```python
from build123d import *

# Parameters (mm, degrees)
F1_DEPTH      = 5.08
F2_START      = -15.494
F2_DEPTH      = 4.826
F3_DEPTH      = 15.748
F3_DEPTH_BACK = 1.016


with BuildPart() as f1:
    # F0 (on Front) → F1 (new body)
    with BuildSketch(Plane.XZ):
        with BuildLine():
            Line((-50.7880747318, 53.6880129844), (-50.7880747318, 47.4713742733))
            Line((-50.7880747318, 47.4713742733), (0, 13.6126577854))
            ThreePointArc((0, 13.6126577854), (30.4237649591, -0.4397436147), (63.6866472612, -4.5209346608))
            Line((63.6866472612, -4.5209346608), (63.7305527925, 0))
            ThreePointArc((63.7305527925, 0), (33.6220207616, 3.8020605731), (5.8134317271, 15.9536753451))
            ThreePointArc((5.8134317271, 15.9536753451), (2.8748778359, 17.8437288794), (0, 19.8292964965))
            Line((0, 19.8292964965), (-50.7880747318, 53.6880129844))
        make_face()
        with BuildLine():
            Line((-50.7880747318, 47.4713742733), (-50.7880747318, -22.5119870156))
            Line((-50.7880747318, -22.5119870156), (63.5119252682, -22.5119870156))
            Line((63.5119252682, -22.5119870156), (63.6866472612, -4.5209346608))
            ThreePointArc((63.6866472612, -4.5209346608), (30.4237649591, -0.4397436147), (0, 13.6126577854))
            Line((0, 13.6126577854), (-50.7880747318, 47.4713742733))
        make_face()
    extrude(amount=F1_DEPTH)



with BuildPart() as f2:
    # F0 (on Front) → F2 (new body)
    with BuildSketch(Plane.XZ.offset(F2_START)):
        with BuildLine():
            Line((-50.7880747318, 47.4713742733), (-50.7880747318, -22.5119870156))
            Line((-50.7880747318, -22.5119870156), (63.5119252682, -22.5119870156))
            Line((63.5119252682, -22.5119870156), (63.6866472612, -4.5209346608))
            ThreePointArc((63.6866472612, -4.5209346608), (30.4237649591, -0.4397436147), (0, 13.6126577854))
            Line((0, 13.6126577854), (-50.7880747318, 47.4713742733))
        make_face()
        with BuildLine():
            Line((-50.7880747318, 53.6880129844), (-50.7880747318, 47.4713742733))
            Line((-50.7880747318, 47.4713742733), (0, 13.6126577854))
            ThreePointArc((0, 13.6126577854), (30.4237649591, -0.4397436147), (63.6866472612, -4.5209346608))
            Line((63.6866472612, -4.5209346608), (63.7305527925, 0))
            ThreePointArc((63.7305527925, 0), (33.6220207616, 3.8020605731), (5.8134317271, 15.9536753451))
            ThreePointArc((5.8134317271, 15.9536753451), (2.8748778359, 17.8437288794), (0, 19.8292964965))
            Line((0, 19.8292964965), (-50.7880747318, 53.6880129844))
        make_face()
        with BuildLine():
            Line((5.8134317271, 15.9536753451), (0, 19.8292964965))
            ThreePointArc((0, 19.8292964965), (2.8748778359, 17.8437288794), (5.8134317271, 15.9536753451))
        make_face()
    extrude(amount=-F2_DEPTH)


with BuildPart() as f1_1:
    add(f1.part)

    add(f2.part)  # F3 merges F2
    # F0 (on Front) → F3 (join, two sides)
    with BuildSketch(Plane.XZ) as f3_sk:
        with BuildLine():
            Line((-50.7880747318, 47.4713742733), (-50.7880747318, -22.5119870156))
            Line((-50.7880747318, -22.5119870156), (63.5119252682, -22.5119870156))
            Line((63.5119252682, -22.5119870156), (63.6866472612, -4.5209346608))
            ThreePointArc((63.6866472612, -4.5209346608), (30.4237649591, -0.4397436147), (0, 13.6126577854))
            Line((0, 13.6126577854), (-50.7880747318, 47.4713742733))
        make_face()
    extrude(amount=-F3_DEPTH)
    extrude(f3_sk.sketch, amount=F3_DEPTH_BACK)


solid = f1_1.part
```
For this review, take the finished solid that the model builds, in its own axes (mm). A direction names the side the tool comes from. Round coordinates to 2 decimals unless told otherwise and drop trailing zeros. Loops run counter-clockwise (first coordinate to the right, second up) from the corner with the lowest first, then second, coordinate; pieces in that order, holes last.
Q1. To check wall thickness, follow line 1 along X through (y, z) = (5, -7); line 2 along X through (y, z) = (7.25, 17); line 3 along Z through (x, y) = (-33.5, 13.5). State the ranges of each line that lie inside material, in increasing order.
Result sheet:
line 1: x = -50.79 to 63.66
line 2: x = -50.79 to -5.08
line 3: z = -22.51 to 35.95
Q2. Add section C-C on z = 44. Write out the cut boundary in (x, y).
Result sheet:
outline: (-50.79, -5.08) - (-36.26, -5.08) - (-36.26, 0) - (-45.58, 0) - (-45.58, 15.49) - (-36.26, 15.49) - (-36.26, 20.32) - (-50.79, 20.32) - close
Q3. Add section D-D on y = 11.25. Write out the cut boundary in (x, z).
Result sheet:
outline: (-50.79, -22.51) - (63.51, -22.51) - (63.69, -4.52) arc R108.33 cw to (0, 13.61) - (-50.79, 47.47) - close
Q4. Insertion check: pin 1 Ø1.5 at (x, y) = (-15, 6.5) entering from +Z; pin 2 Ø6 at (y, z) = (17, 40.5) entering from +X; pin 3 Ø1.5 at (y, z) = (14.5, 11) entering from +X. Each pin has a flat end and moves straight along its axis. Give the tip position at first contact, or say it passes through.
Result sheet:
pin 1: stops at z = 24.11
pin 2: stops at x = -26.51
pin 3: stops at x = 5.38
Q5. Add section B-B on x = -34. Write out the cut boundary in (y, z), plus the area to 3 significant figures.
Result sheet:
outline: (-5.08, -22.51) - (20.32, -22.51) - (20.32, 42.5) - (15.49, 42.5) - (15.49, 36.28) - (0, 36.28) - (0, 42.5) - (-5.08, 42.5) - close
area: 1,550 mm2
Q6. Machinability: for faces 1 (the face through (2, 15.494, 18)), 2 (the face through (6, 8, -22.512)), which of the approach directions +Z, -Z, +X, -X, +Y, -Y give a long, thin tool a straight path to every point of the face, cutting with its end or side? Answer none if there is none.
Result sheet:
face 1: +Z, +X
face 2: -Z, +X, -X, +Y, -Y
Q7. Add section A-A on y = 18.75. Write out the cut boundary in (x, z).
Result sheet:
outline: (-50.79, -22.51) - (63.51, -22.51) - (63.73, 0) arc R106.34 cw to (5.81, 15.95) - (-50.79, 53.69) - close
